from build123d import *

# Parameters (mm, degrees)
CROQUIS2_R              = 0.5
SALIENTE_EXTRUIR1_DEPTH = 1.5
CROQUIS3_R              = 4.5
SALIENTE_EXTRUIR2_DEPTH = 2.3
CROQUIS4_R              = 3
CORTAR_EXTRUIR1_DEPTH   = 0.9
CROQUIS5_R              = 1.5
CORTAR_EXTRUIR2_DEPTH   = 21.730533037
CROQUIS6_R              = 2.7
CORTAR_EXTRUIR3_DEPTH   = 2.5


with BuildPart() as part:
    # Croquis2 → Saliente-Extruir1 (new body)
    with BuildSketch(Plane(origin=(0, 0, 0), x_dir=(1, 0, 0), z_dir=(0, 1, 0))):
        with BuildLine():
            Line((2.6, 16.75), (4.7, 4.983221849))
            ThreePointArc((4.7, 4.983221849), (6.85, 0), (4.7, -4.983221849))
            Line((4.7, -4.983221849), (2.6, -16.75))
            ThreePointArc((2.6, -16.75), (0, -19.35), (-2.6, -16.75))
            Line((-2.6, -16.75), (-4.7, -4.983221849))
            ThreePointArc((-4.7, -4.983221849), (-6.85, 0), (-4.7, 4.983221849))
            Line((-4.7, 4.983221849), (-2.6, 16.75))
            ThreePointArc((-2.6, 16.75), (0, 19.35), (2.6, 16.75))
        make_face()
        with Locations(Location((0, -16.5, 0), (0, 0, 90))):
            Circle(CROQUIS2_R, mode=Mode.SUBTRACT)
        with Locations(Location((0, -13.5, 0), (0, 0, 90))):
            Circle(CROQUIS2_R, mode=Mode.SUBTRACT)
        with Locations(Location((0, -10.5, 0), (0, 0, 90))):
            Circle(CROQUIS2_R, mode=Mode.SUBTRACT)
        with Locations(Location((0, -7.5, 0), (0, 0, 90))):
            Circle(CROQUIS2_R, mode=Mode.SUBTRACT)
        with Locations(Location((0, 7.5, 0), (0, 0, 270))):
            Circle(CROQUIS2_R, mode=Mode.SUBTRACT)
        with Locations(Location((0, 10.5, 0), (0, 0, 270))):
            Circle(CROQUIS2_R, mode=Mode.SUBTRACT)
        with Locations(Location((0, 13.5, 0), (0, 0, 270))):
            Circle(CROQUIS2_R, mode=Mode.SUBTRACT)
        with Locations(Location((0, 16.5, 0), (0, 0, 270))):
            Circle(CROQUIS2_R, mode=Mode.SUBTRACT)
    extrude(amount=SALIENTE_EXTRUIR1_DEPTH)

    # Croquis3 → Saliente-Extruir2 (add)
    with BuildSketch(Plane(origin=(0, 1.5, 0), x_dir=(1, 0, 0), z_dir=(0, 1, 0))):
        with Locations(Location((0, 0, 0), (0, 0, 270))):
            Circle(CROQUIS3_R)
    extrude(amount=SALIENTE_EXTRUIR2_DEPTH)

    # Croquis4 → Cortar-Extruir1 (cut)
    with BuildSketch(Plane.XZ):
        with Locations(Location((0, 0, 0), (0, 0, 270))):
            Circle(CROQUIS4_R)
    extrude(amount=-CORTAR_EXTRUIR1_DEPTH, mode=Mode.SUBTRACT)

    # Croquis5 → Cortar-Extruir2 (cut, through all)
    with BuildSketch(Plane.XZ.offset(-0.9)):
        with Locations(Location((0, 0, 0), (0, 0, 270))):
            Circle(CROQUIS5_R)
    extrude(amount=-CORTAR_EXTRUIR2_DEPTH, mode=Mode.SUBTRACT)

    # Croquis6 → Cortar-Extruir3 (cut)
    with BuildSketch(Plane(origin=(0, 3.8, 0), x_dir=(1, 0, 0), z_dir=(0, 1, 0))):
        with Locations(Location((0, 0, 0), (0, 0, 270))):
            Circle(CROQUIS6_R)
    extrude(amount=-CORTAR_EXTRUIR3_DEPTH, mode=Mode.SUBTRACT)


solid = part.part
CAD build for the part. Positions are in the model's coordinates, mm. A direction names the side the tool comes from. Give positions to 0.01 mm unless a question says otherwise; leave off trailing zeros. Order: outer loops, then holes, each group sorted by start corner. A loop starts at its lowest first (then second) coordinate and runs counter-clockwise, first axis right, second up. Notation, with made-up numbers: (55, 14) -> (75, 14) arc R19 cw to (75, 31) -> close; hole circle Ø6 at (40, -20). An arc over 180 degrees is marked (long way). Return JSON: item names as keys, results as strings.
Q1. Drill centre lines: line 1 (Y direction, x = 1.75, z = -14.5); line 2 (Z direction, x = -1, y = 2.9); line 3 (X direction, y = 0.8, z = 10.5). Where is each one in solid material? Low to high.
Working result:
{"line 1": "0 to 1.5", "line 2": "-4.39 to -2.51, 2.51 to 4.39", "line 3": "-3.72 to -0.5, 0.5 to 3.72"}
Q2. Which spindle directions (+Z, -Z, +X, -X, +Y, -Y) get a long thin tool onto all of the face, cutting with end or side? Do faces 4 (the face through (0, 1, 7)), 5 (the face through (0.811, 2.568, 2.575)), 6 (the face through (-1.3, 0.9, -1.3)). Say none if no direction does.
Working result:
{"face 4": "+Y, -Y", "face 5": "+Y", "face 6": "-Y"}
Q3. Mould opens along Z. For faces 1 (the face through (-3, 3.8, 0)), 2 (the face through (3.665, 0.74, 10.784)), 3 (the face through (0, 1, -11)) say: pulls with the +Z half, pulls with the -Z half, needs draft (parallel to the pull), parting line crosses it, or undercut.
Working result:
{"face 1": "needs draft", "face 2": "pulls with the +Z half", "face 3": "undercut"}
Q4. Flat gauge pins, fed straight in: pin 1 (1.8 mm diameter, centred on x = 0, z = 0, fed in from +Y); pin 2 (4.5 mm diameter, centred on x = -0.5, z = 0.5, fed in from +Y); pin 3 (2 mm diameter, centred on x = 2, y = 0.5, fed in from +Z); pin 4 (1.5 mm diameter, centred on y = 1.5, z = -2, fed in from -X) (3 decimals). Where does each tip first touch, or does it go through?
Working result:
{"pin 1": "through", "pin 2": "y = 3.8", "pin 3": "z = 19.15", "pin 4": "x = -6.735"}
Q5. Saw through at D-D (z = 7.5). Write the cut outline in (x, y), then the cut area to 3 significant figures.
Working result:
{"outline": "(-4.25, 0) -> (-0.5, 0) -> (-0.5, 1.5) -> (-4.25, 1.5) -> close; (0.5, 0) -> (4.25, 0) -> (4.25, 1.5) -> (0.5, 1.5) -> close", "area": "11.3 mm²"}
Q6. Saw through at C-C (y = 3.4). Write the cut outline in (x, z).
Working result:
{"outline": "circle Ø9 at (0, 0); hole circle Ø5.4 at (0, 0)"}
Q7. Saw through at A-A (z = 0). Write the cut outline in (x, y).
Working result:
{"outline": "(-6.85, 0) -> (-3, 0) -> (-3, 0.9) -> (-1.5, 0.9) -> (-1.5, 1.3) -> (-2.7, 1.3) -> (-2.7, 3.8) -> (-4.5, 3.8) -> (-4.5, 1.5) -> (-6.85, 1.5) -> close; (1.5, 0.9) -> (3, 0.9) -> (3, 0) -> (6.85, 0) -> (6.85, 1.5) -> (4.5, 1.5) -> (4.5, 3.8) -> (2.7, 3.8) -> (2.7, 1.3) -> (1.5, 1.3) -> close"}
Q8. Saw through at B-B (x = 0). Count the separate pieces of the cut face and the enclosed holes in it, then the cut area to 4 significant figures.
Working result:
{"separate pieces": "10", "enclosed holes": "0", "area": "46.65 mm²"}
